Verification items for the finished model (mm, model axes). A direction names the side the tool comes from. Round coordinates to 2 decimals unless told otherwise and drop trailing zeros. Order: outer loops, then holes, each group sorted by start corner. A loop starts at its lowest first (then second) coordinate and runs counter-clockwise, first axis right, second up. Notation, with made-up numbers: (29, 56) -> (72, 56) arc R20 ccw to (72, 69) -> close; hole circle Ø1 at (87.5, 67.5). An arc over 180 degrees is marked (long way). Put each result on its own line as item: value.
Autodesk Inventor part; units mm, degrees
ref_plane "YZ Plane" through (0, 0, 0) normal (1, 0, 0) x (0, 1, 0)
ref_plane "XZ Plane" through (0, 0, 0) normal (0, 1, 0) x (-1, 0, 0)
ref_plane "XY Plane" through (0, 0, 0) normal (0, 0, 1) x (1, 0, 0)
sketch "Sketch1" plane through (0, 0, 0) normal (0, 0, 1) x (1, 0, 0)
  circle A0 centre (0, 0) radius 2.5
  circle A1 centre (0, 0) radius 7.5
  line L0 (-7.5, 0) -> (112.5, 0)
  line L1 (112.5, 0) -> (112.5, 7.5)
  line L2 (112.5, 7.5) -> (-7.5, 7.5)
  line L3 (-7.5, 7.5) -> (-7.5, 0)
  circle A2 centre (105, 0) radius 7.5 construction
  circle A3 centre (105, 0) radius 2
  line L4 (112.5, 7.5) -> (105, 7.5)
  line L5 (105, 7.5) -> (105, -7.5)
  line L6 (105, -7.5) -> (112.5, -7.5)
  line L7 (112.5, -7.5) -> (112.5, 7.5)
  circle A4 centre (116, 4) radius 3.5
  line L8 (112.5, 7.5) -> (116, 7.5)
  arc A5 (117.6076, 0.891) -> (112.5, -7.5) centre (121.9464, -7.5) ccw
  point P0 (7.5, 0)
  point P1 (103, 0)
  point P2 (105, -2)
  dimension "d1" = 15
  dimension "d3" = 15
  dimension "d0" = 5
  dimension "d2" = 120
  dimension "d4" = 4
  dimension "d5" = 7
extrude "Extrusion1" add sketch "Sketch1" along normal blind 15 contours L0 A1 A0 | A0 L0 A1 | A1 L2 L5 A3 L0 | L3 L2 A1 | L2 L1 L0 A3 L5 | A3 L0 L7 L6 L5 | L8 A4 L1 | A4 A5 L7 L1 | A4
fillet "Fillet1" radius 2 5 edges at (103, 0, 7.5) (105, -2, 7.5) (105, -7.5, 7.5) (112.5, -7.5, 7.5) (7.5, 0, 7.5)
fillet "Fillet2" radius 5 1 edges at (-7.5, 7.5, 7.5)
properties part number "Lid"
Item 1: Depth check by flat-ended pin: pin 1 Ø1.6 at (y, z) = (-5, 5) entering from -X; pin 2 Ø1.5 at (x, z) = (89.5, 1.5) entering from -Y. Enter the tip coordinate at first touch or a pass-through.
Geometry check:
pin 1: x = -6.21
pin 2: y = 0
Item 2: Release check for a two-part mould opening along X. For faces 1 (the face through (-0.641, -7.473, 7.395)), 2 (the face through (112, -7, 8)), 3 (the face through (109, -7.5, 7)) record: pulls with the +X half, pulls with the -X half, needs draft (parallel to the pull), parting line crosses it, or undercut.
Geometry check:
face 1: undercut
face 2: pulls with the +X half
face 3: needs draft
Item 3: Sectioned sample at A-A, the plane z = 9. Record the boundary of the cut face in (x, y).
Geometry check:
outline: (-7.5, 0) arc R7.5 ccw to (7.33, -1.58) arc R2 cw to (9.29, 0) -> (101.54, 0) arc R2 ccw to (103.27, 1) arc R2 cw (long way) to (106, -1.73) arc R2 ccw to (105, -3.46) -> (105, -5.5) arc R2 ccw to (107, -7.5) -> (110.68, -7.5) arc R2 ccw to (112.65, -5.85) arc R9.45 cw to (117.61, 0.89) arc R3.5 ccw to (116, 7.5) -> (-2.5, 7.5) arc R5 ccw to (-7.5, 2.5) -> close; hole circle Ø5 at (0, 0)
Item 4: Material ranges on line 1 along X through (y, z) = (-1, 13.75); line 2 along Y through (x, z) = (48.5, 5); line 3 along X through (y, z) = (-3.25, 2.5), recorded low to high.
Geometry check:
line 1: -7.43 to -2.29, 2.29 to 7.56, 106.73 to 115.09
line 2: 0 to 7.5
line 3: -6.76 to 6.76, 105.01 to 113.51
Item 5: Tool access check on faces 4 (the face through (105, -4, 7)), 5 (the face through (-7.5, 1, 7)). Record the directions out of +Z, -Z, +X, -X, +Y, -Y that give a thin tool (end or side, any length) a straight path to the whole face; none if there is none.
Geometry check:
face 4: +Z, -Z, -Y
face 5: +Z, -Z, -X, +Y, -Y
Item 6: Sectioned sample at B-B, the plane x = 99. Record the boundary of the cut face in (y, z).
Geometry check:
outline: (0, 0) -> (7.5, 0) -> (7.5, 15) -> (0, 15) -> close
